Work out the finished part from the listing and answer in its coordinate system (mm). Round coordinates to 2 decimals unless told otherwise and drop trailing zeros. Write each loop counter-clockwise with the first axis right and the second up, starting at its lowest first coordinate (ties: lowest second). Pieces come first, ordered by that corner, then holes. Notation, with made-up numbers: M 74,49 L 98,49 A31 ccw 98,77 Z; hole C -9,-39 d5. An arc over 180 degrees is marked long. Answer in a Markdown table with one row per item.
```python
from build123d import *

# Parameters (mm, degrees)
SKETCH1_R           = 22
SKETCH1_R_2         = 18
BOSS_EXTRUDE1_DEPTH = 6
BOSS_EXTRUDE2_DEPTH = 6
CUT_EXTRUDE1_DEPTH  = 37.933063475
SKETCH4_W           = 4
SKETCH4_H           = 30
BOSS_EXTRUDE3_DEPTH = 6
CUT_EXTRUDE2_DEPTH  = 57.332617611
FILLET1_R           = 20
FILLET2_R           = 20
SKETCH6_W           = 4
SKETCH6_H           = 120
BOSS_EXTRUDE4_DEPTH = 6
BOSS_EXTRUDE5_DEPTH = 6
FILLET3_R           = 3


with BuildPart() as part:
    # Sketch1 → Boss-Extrude1 (new body)
    with BuildSketch(Plane(origin=(0, 0, 0), x_dir=(0, 0, -1), z_dir=(1, 0, 0))):
        Circle(SKETCH1_R)
        Circle(SKETCH1_R_2, mode=Mode.SUBTRACT)
    extrude(amount=BOSS_EXTRUDE1_DEPTH)

    # Sketch2 → Boss-Extrude2 (add)
    with BuildSketch(Plane(origin=(6, 0, 0), x_dir=(0, 0, -1), z_dir=(1, 0, 0))):
        Polygon((19.052558883, 11), (29.052558883, -6.320508076), (25.588457268, -8.320508076), (15.588457268, 9), align=None)
    extrude(amount=-BOSS_EXTRUDE2_DEPTH)

    # Sketch3 → Cut-Extrude1 (cut, through all)
    with BuildSketch(Plane(origin=(6, 0, 0), x_dir=(0, 0, -1), z_dir=(1, 0, 0))):
        with BuildLine():
            ThreePointArc((18, 0), (14.280360125, -10.957705722), (4.658742812, -17.386664873))
            Line((4.658742812, -17.386664873), (5.694018992, -21.250368178))
            ThreePointArc((5.694018992, -21.250368178), (16.84102585, -14.15555892), (21.913012588, -1.95445115))
            Line((21.913012588, -1.95445115), (15.588457268, 9))
            ThreePointArc((15.588457268, 9), (17.386664873, 4.658742812), (18, 0))
        make_face()
    extrude(amount=-CUT_EXTRUDE1_DEPTH, mode=Mode.SUBTRACT)

    # Sketch4 → Boss-Extrude3 (add)
    with BuildSketch(Plane(origin=(6, 0, 0), x_dir=(0, 0, -1), z_dir=(1, 0, 0))):
        with Locations((0, -32.88854382)):
            Rectangle(SKETCH4_W, SKETCH4_H)
    extrude(amount=-BOSS_EXTRUDE3_DEPTH)

    # Sketch5 → Cut-Extrude2 (cut, through all)
    with BuildSketch(Plane(origin=(6, 0, 0), x_dir=(0, 0, -1), z_dir=(1, 0, 0))):
        with BuildLine():
            Line((2, -21.9089023), (2, -17.88854382))
            Line((2, -17.88854382), (4.658742812, -17.386664873))
            Line((4.658742812, -17.386664873), (5.694018992, -21.250368178))
            ThreePointArc((5.694018992, -21.250368178), (3.876129227, -21.742981124), (2, -21.9089023))
        make_face()
    extrude(amount=-CUT_EXTRUDE2_DEPTH, mode=Mode.SUBTRACT)

    # Fillet1
    # the kernel refuses this fillet: 20 mm, written as the material it adds along each edge
    with BuildSketch(Plane(origin=(6, -21.9089023, 2), x_dir=(0, -1, 0), z_dir=(-1, 0, 0))) as fillet1_piece_1:
        with BuildLine():
            CenterArc((13.86818534, 20), FILLET1_R, 211.588135505, 58.411864495)
            ThreePointArc((-3.16852306, 9.523809524), (-1.033875129, 4.945015522), (0, 0))
            Line((0, 0), (13.86818534, 0))
        make_face()
    extrude(amount=6)
    # the kernel refuses this fillet: 20 mm, written as the material it takes off along each edge
    with BuildSketch(Plane(origin=(36, -17.88854382, -2), x_dir=(0, -1, 0), z_dir=(-1, 0, 0))) as fillet1_2_piece_1:
        with BuildLine():
            CenterArc((12, 20), FILLET1_R, 233.130102354, 36.869897646)
            Line((0, 4), (0, 0))
            Line((0, 0), (12, 0))
        make_face()
    extrude(amount=66, mode=Mode.SUBTRACT)

    # Fillet2
    fillet2_edges = [part.edges().sort_by_distance(p)[0] for p in [
        (3, -17.88854382, 2),
    ]]
    fillet(fillet2_edges, radius=FILLET2_R)

    # Sketch6 → Boss-Extrude4 (add)
    with BuildSketch(Plane.ZY):
        with Locations((0, -107.88854382)):
            Rectangle(SKETCH6_W, SKETCH6_H)
    extrude(amount=-BOSS_EXTRUDE4_DEPTH)

    # Sketch7 → Boss-Extrude5 (add)
    with BuildSketch(Plane(origin=(0, 0, -2), x_dir=(0, 0, -1), z_dir=(1, 0, 0))):
        Polygon((-4, -167.88854382), (-22.115183313, -145.397653808), (-19, -142.88854382), (-4, -161.511780713), align=None)
        Polygon((-4, -115.135017606), (-4, -121.511780713), (-22.115183313, -99.0208907), (-19, -96.511780713), align=None)
        Polygon((-4, -68.758254499), (-4, -75.135017606), (-22.115183313, -52.644127593), (-19, -50.135017606), align=None)
    boss_extrude5 = extrude(amount=BOSS_EXTRUDE5_DEPTH)

    # Mirror1: Boss-Extrude5 across plane
    add(boss_extrude5.mirror(Plane.XY))

    # Fillet3
    # the kernel refuses this fillet: 3 mm, written as the material it adds along each edge
    with BuildSketch(Plane(origin=(0, -161.511780713, 2), x_dir=(0, 1, 0), z_dir=(1, 0, 0)), Plane(origin=(0, -115.135017606, 2), x_dir=(0, 1, 0), z_dir=(1, 0, 0)), Plane(origin=(0, -68.758254499, 2), x_dir=(0, 1, 0), z_dir=(1, 0, 0))) as fillet3_piece_1:
        with BuildLine():
            CenterArc((FILLET3_R * 2.83573990297, FILLET3_R), FILLET3_R, 128.849545597, 141.150454403)
            Line((FILLET3_R * 2.20846240609, FILLET3_R * 1.77879582813), (0, 0))
            Line((0, 0), (FILLET3_R * 2.83573990297, 0))
        make_face()
    extrude(amount=6)
    with BuildSketch(Plane(origin=(0, -121.511780713, 2), x_dir=(0, 0.7787958281290415, 0.6272774968774191), z_dir=(1, 0, 0)), Plane(origin=(0, -75.135017606, 2), x_dir=(0, 0.7787958281290404, 0.6272774968774205), z_dir=(1, 0, 0)), Plane(origin=(0, -121.511780713, -2), x_dir=(0, -1, 0), z_dir=(1, 0, 0)), Plane(origin=(0, -75.135017606, -2), x_dir=(0, -1, 0), z_dir=(1, 0, 0))) as fillet3_piece_2:
        with BuildLine():
            CenterArc((FILLET3_R * 0.352641650581, FILLET3_R), FILLET3_R, 231.150454403, 38.849545597)
            Line((-FILLET3_R * 0.274635846297, FILLET3_R * 0.221204171871), (0, 0))
            Line((0, 0), (FILLET3_R * 0.352641650581, 0))
        make_face()
    extrude(amount=6)
    with BuildSketch(Plane(origin=(0, -161.511780713, -2), x_dir=(0, 1, 0), z_dir=(1, 0, 0)), Plane(origin=(0, -115.135017606, -2), x_dir=(0, 1, 0), z_dir=(1, 0, 0)), Plane(origin=(0, -68.758254499, -2), x_dir=(0, 1, 0), z_dir=(1, 0, 0))) as fillet3_piece_3:
        with BuildLine():
            CenterArc((FILLET3_R * 2.83573990297, -FILLET3_R), FILLET3_R, 90, 141.150454403)
            Line((FILLET3_R * 2.20846240609, -FILLET3_R * 1.77879582813), (0, 0))
            Line((0, 0), (FILLET3_R * 2.83573990297, 0))
        make_face()
    extrude(amount=6)
    # the kernel refuses this fillet: 3 mm, written as the material it takes off along each edge
    with BuildSketch(Plane(origin=(-3.589411592, -167.88854382, 2), x_dir=(0, 0.7787958281290398, 0.6272774968774211), z_dir=(1, 0, 0)), Plane(origin=(-3.589411592, -167.88854382, -2), x_dir=(0, 0, 1), z_dir=(1, 0, 0))) as fillet3_2_piece_1:
        with BuildLine():
            CenterArc((FILLET3_R * 0.478588212289, -FILLET3_R), FILLET3_R, 90, 51.150454403)
            Line((-FILLET3_R * 0.30020761584, -FILLET3_R * 0.372722503123), (0, 0))
            Line((0, 0), (FILLET3_R * 0.478588212289, 0))
        make_face()
    extrude(amount=13.178823184, mode=Mode.SUBTRACT)
    with BuildSketch(Plane(origin=(-7.5, -145.397653808, 20.115183313), x_dir=(0, 0.6272774968774232, -0.7787958281290382), z_dir=(1, 0, 0)), Plane(origin=(-7.5, -99.0208907, 20.115183313), x_dir=(0, 0.6272774968774221, -0.7787958281290391), z_dir=(1, 0, 0)), Plane(origin=(-7.5, -52.644127593, 20.115183313), x_dir=(0, 0.6272774968774235, -0.778795828129038), z_dir=(1, 0, 0)), Plane(origin=(-7.5, -145.397653808, -20.115183313), x_dir=(0, -0.7787958281290382, 0.627277496877423), z_dir=(1, 0, 0)), Plane(origin=(-7.5, -99.0208907, -20.115183313), x_dir=(0, -0.7787958281290382, 0.627277496877423), z_dir=(1, 0, 0)), Plane(origin=(-7.5, -52.644127593, -20.115183313), x_dir=(0, -0.7787958281290385, 0.6272774968774228), z_dir=(1, 0, 0))) as fillet3_2_piece_2:
        with BuildLine():
            CenterArc((FILLET3_R, -FILLET3_R), FILLET3_R, 90, 90)
            Line((0, -FILLET3_R), (0, 0))
            Line((0, 0), (FILLET3_R, 0))
        make_face()
    extrude(amount=21, mode=Mode.SUBTRACT)
    with BuildSketch(Plane(origin=(13.5, -8.320508076, -25.588457268), x_dir=(0, 0.8660254037844379, 0.5000000000000012), z_dir=(-1, 0, 0)), Plane(origin=(13.5, -6.320508076, -29.052558883), x_dir=(0, -0.5000000000000019, 0.8660254037844376), z_dir=(-1, 0, 0))) as fillet3_2_piece_3:
        with BuildLine():
            CenterArc((FILLET3_R, FILLET3_R), FILLET3_R, 180, 90)
            Line((0, FILLET3_R), (0, 0))
            Line((0, 0), (FILLET3_R, 0))
        make_face()
    extrude(amount=21, mode=Mode.SUBTRACT)


solid = part.part
```
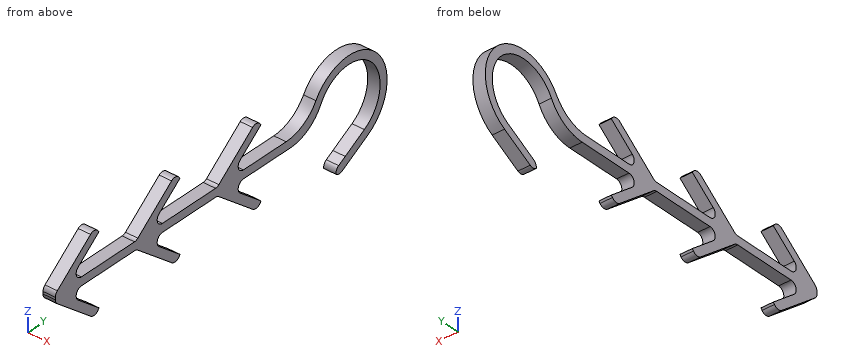
1. Given pin 1 (5 mm diameter, centred on y = -104.5, z = 5, fed in from -X); pin 2 (3 mm diameter, centred on x = 2, y = -44.5, fed in from -Z); pin 3 (3 mm diameter, centred on x = 1, z = -2.5, fed in from +Y); pin 4 (3 mm diameter, centred on x = 3, z = 10.5, fed in from -Y), each flat-ended and moving along its own axis, determine where each tip first touches the part or whether it passes through.
Calculated:
| item | result |
|---|---|
| pin 1 | passes through |
| pin 2 | stops at z = -2 |
| pin 3 | stops at y = 21.98 |
| pin 4 | stops at y = -159.2 |
2. Consider line 1 along Y through (x, z) = (4, -11); line 2 along Y through (x, z) = (1.25, -3); line 3 along Y through (x, z) = (4, 4.5). Determine where each line is inside the solid, lowest interval first. Write a range as from..to.
Calculated:
| item | result |
|---|---|
| line 1 | y = -156.71..-150.34, -110.34..-103.96, -63.96..-57.58, 14.25..19.05 |
| line 2 | y = -166.65..-155.24, -120.27..-108.86, -73.89..-62.49, 17.75..21.79 |
| line 3 | y = -164.78..-155.96, -118.41..-109.59, -72.03..-63.21, -26.09..-18.71, 17.43..21.53 |
3. The part is cut by section A-A (y = 0). Determine the outline of the cut face in (x, z).
Calculated:
| item | result |
|---|---|
| outline | M 0,-25.4 L 6,-25.4 L 6,-20.78 L 0,-20.78 Z; M 0,18 L 6,18 L 6,22 L 0,22 Z |
4. The part is cut by section B-B (z = -13.5). Determine the outline of the cut face in (x, y), plus the area to 3 significant figures.
Calculated:
| item | result |
|---|---|
| outline | M 0,-153.61 L 6,-153.61 L 6,-147.23 L 0,-147.23 Z; M 0,-107.23 L 6,-107.23 L 6,-100.86 L 0,-100.86 Z; M 0,-60.86 L 6,-60.86 L 6,-54.48 L 0,-54.48 Z; M 0,11.91 L 6,11.91 L 6,17.37 L 0,17.37 Z |
| area | 148 mm² |
